Input: dimensioned drawing with shaded views. Units: mm. Origin: part minimum x, y, z. A direction names the side the tool comes from. Coordinates: 2 decimals unless noted, no trailing zeros. Order: outer loops, then holes, each group sorted by start corner. A loop starts at its lowest first (then second) coordinate and runs counter-clockwise, first axis right, second up. Notation, with made-up numbers: (-4, 0.5) -> (35, 0.5) arc R16 cw to (35, 9.5) -> close; hole circle Ø3 at (16, -32). An arc over 180 degrees is marked (long way). Put each result on its own line as item: value.
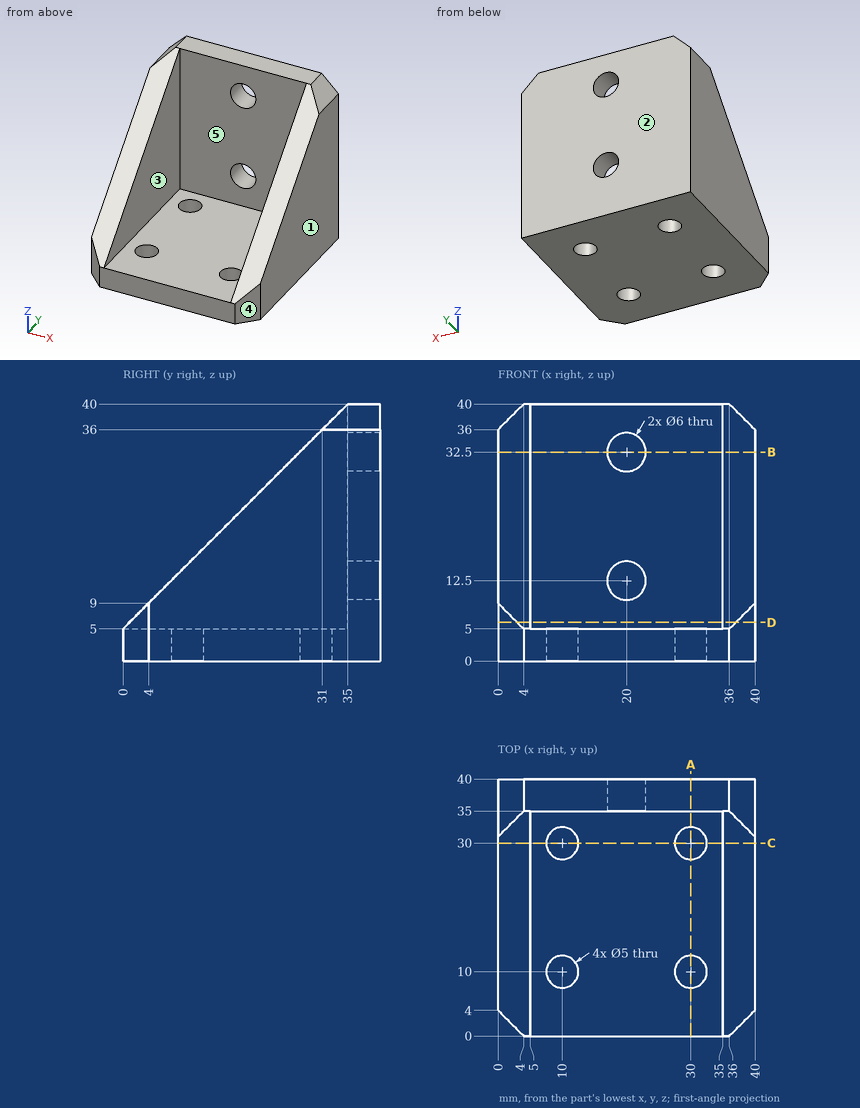
1. Cut plane D-D on z = 6. Output: boundary loops of the cut face in (x, y), plus the area to 3 significant figures.
Numbers:
outline: (0, 4) -> (3, 1) -> (5, 1) -> (5, 35) -> (35, 35) -> (35, 1) -> (37, 1) -> (40, 4) -> (40, 40) -> (0, 40) -> close
area: 531 mm2
2. Cut plane B-B on z = 32.5. Output: boundary loops of the cut face in (x, y), plus the area to 3 significant figures.
Numbers:
outline: (0, 27.5) -> (5, 27.5) -> (5, 35) -> (17, 35) -> (17, 40) -> (0, 40) -> close; (23, 35) -> (35, 35) -> (35, 27.5) -> (40, 27.5) -> (40, 40) -> (23, 40) -> close
area: 245 mm2
3. First-contact query: pin 1 (6 mm diameter, centred on x = 10, y = 10, fed in from +Z); pin 2 (12 mm diameter, centred on x = 16, z = 31, fed in from -Y). Flat tips, straight axial feed; report the tip coordinate or a pass-through.
Numbers:
pin 1: stops at z = 5
pin 2: stops at y = 35
4. Cut plane C-C on y = 30. Output: boundary loops of the cut face in (x, z), plus the area to 3 significant figures.
Numbers:
outline: (0, 0) -> (7.5, 0) -> (7.5, 5) -> (5, 5) -> (5, 35) -> (0, 35) -> close; (12.5, 0) -> (27.5, 0) -> (27.5, 5) -> (12.5, 5) -> close; (32.5, 0) -> (40, 0) -> (40, 35) -> (35, 35) -> (35, 5) -> (32.5, 5) -> close
area: 450 mm2
5. Cut plane A-A on x = 30. Output: boundary loops of the cut face in (y, z).
Numbers:
outline: (0, 0) -> (7.5, 0) -> (7.5, 5) -> (0, 5) -> close; (12.5, 0) -> (27.5, 0) -> (27.5, 5) -> (12.5, 5) -> close; (32.5, 0) -> (40, 0) -> (40, 40) -> (35, 40) -> (35, 5) -> (32.5, 5) -> close
6. Ray query, line 1 along Y through (x, z) = (30, 3.7); line 2 along X through (y, z) = (10, 14); line 3 along Z through (x, y) = (20, 38.2). Return the intervals inside material, ascending.
Numbers:
line 1: y = 0 to 7.5, 12.5 to 27.5, 32.5 to 40
line 2: x = 0 to 5, 35 to 40
line 3: z = 0 to 9.5, 15.5 to 29.5, 35.5 to 40
7. Pull-direction query (X, two-part tool) for the marked faces 1, 2 and 3; classes: pulls with the +X half, pulls with the -X half, needs draft (parallel to the pull), parting line crosses it, or undercut.
Numbers:
face 1: pulls with the +X half
face 2: needs draft
face 3: undercut
8. Set-up query: the marked faces 4 and 5. Return all of +Z, -Z, +X, -X, +Y, -Y with unobstructed straight access to the full face (end or side cutting, diameter ignored); none if empty.
Numbers:
face 4: +Z, -Z, +X, -Y
face 5: +Z, -Y
